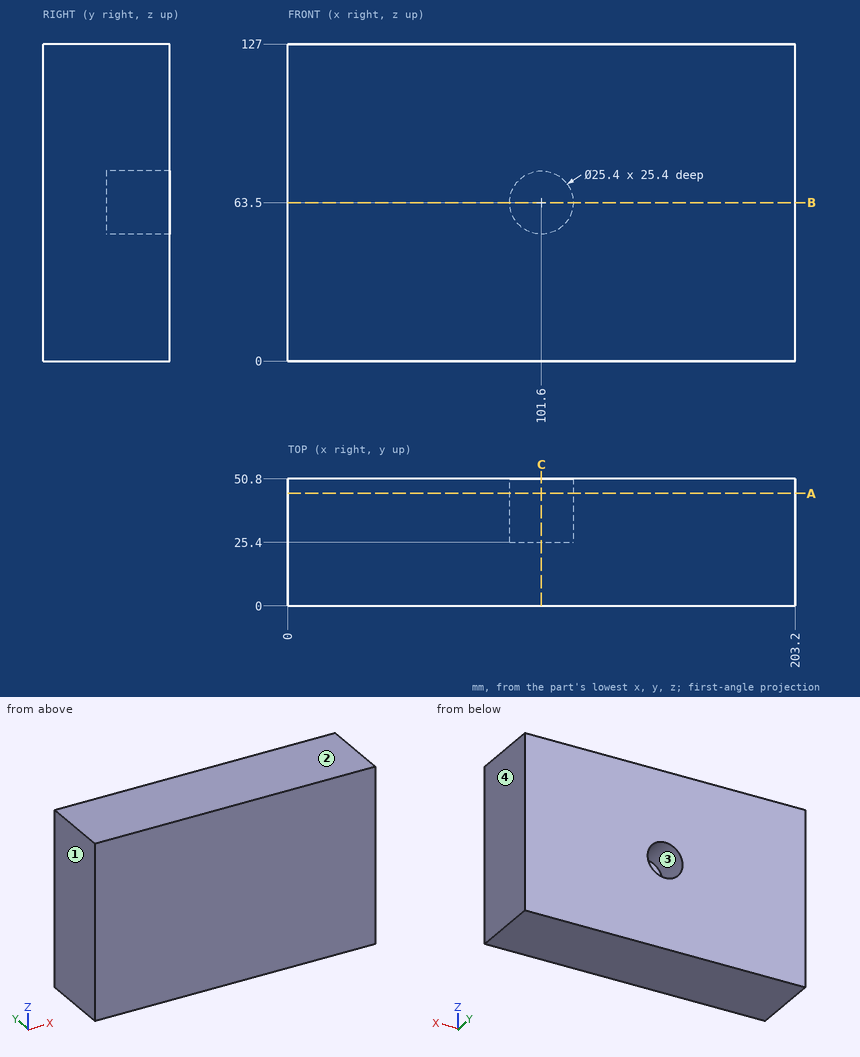
Part print with two shaded views. Sizes in mm from the minimum x, y, z corner. Coordinates: 2 decimals unless noted, no trailing zeros. Write each loop counter-clockwise with the first axis right and the second up, starting at its lowest first coordinate (ties: lowest second). Pieces come first, ordered by that corner, then holes. Notation, with made-up numbers: (64, 79.25) - (75, 79.25) arc R22 cw to (75, 108.25) - close; hole circle Ø3 at (20, 82.25). An arc over 180 degrees is marked (long way). One line per item, written item: value. Start each with the question number.
1. Slice it at A-A (y = 45). Write the cut outline in (x, z), plus the area to 3 significant figures.
2. Probe line 1 (Z direction, x = 101.6, y = 44.25); line 2 (X direction, y = 39, z = 63); line 3 (Y direction, x = 95.5, z = 72.5). List the from-to ranges inside material, lowest first. Write a range as from..to.
3. Slice it at C-C (x = 101.6). Write the cut outline in (y, z).
4. Slice it at B-B (z = 63.5). Write the cut outline in (x, y).
5. Mould opens along X. For the marked faces 1, 2, 3 and 4 say: released by +X, released by -X, zero draft, split by the parting line, or undercut.
Answers below:
1. outline: (0, 0) - (203.2, 0) - (203.2, 127) - (0, 127) - close; hole circle Ø25.4 at (101.6, 63.5)
1. area: 25,300 mm^2
2. line 1: z = 0..50.8, 76.2..127
2. line 2: x = 0..88.91, 114.29..203.2
2. line 3: y = 0..25.4
3. outline: (0, 0) - (50.8, 0) - (50.8, 50.8) - (25.4, 50.8) - (25.4, 76.2) - (50.8, 76.2) - (50.8, 127) - (0, 127) - close
4. outline: (0, 0) - (203.2, 0) - (203.2, 50.8) - (114.3, 50.8) - (114.3, 25.4) - (88.9, 25.4) - (88.9, 50.8) - (0, 50.8) - close
5. face 1: released by -X
5. face 2: zero draft
5. face 3: undercut
5. face 4: released by +X
